from build123d import *

# Parameters (mm, degrees)
F0_W     = 30
F0_H     = 30
F0_W_2   = 25.6
F0_H_2   = 25.6
F1_DEPTH = 200
F2_R     = 3.1
F3_DEPTH = 35
F4_R     = 3.1
F5_DEPTH = 35


with BuildPart() as f1:
    # F0 (on Front) → F1 (new body)
    with BuildSketch(Plane.XZ):
        with Locations((15, 15)):
            Rectangle(F0_W, F0_H)
        with Locations((15, 15)):
            Rectangle(F0_W_2, F0_H_2, mode=Mode.SUBTRACT)
    extrude(amount=F1_DEPTH)

    # F2 (on face) → F3 (cut)
    with BuildSketch(Plane.XY.offset(30)):
        with Locations((15, -20)):
            Circle(F2_R)
        with Locations((15, -100)):
            Circle(F2_R)
        with Locations((15, -180)):
            Circle(F2_R)
    extrude(amount=-F3_DEPTH, mode=Mode.SUBTRACT)

    # F4 (on face) → F5 (cut)
    with BuildSketch(Plane.YZ.offset(30)):
        with Locations((-166.5, 15)):
            Circle(F4_R)
        with Locations((-33.5, 15)):
            Circle(F4_R)
    extrude(amount=-F5_DEPTH, mode=Mode.SUBTRACT)


solid = f1.part
Work out the finished part from the listing and answer in its coordinate system (mm). A direction names the side the tool comes from. Coordinates: 2 decimals unless noted, no trailing zeros. Write each loop counter-clockwise with the first axis right and the second up, starting at its lowest first coordinate (ties: lowest second). Pieces come first, ordered by that corner, then holes. Notation, with made-up numbers: M -14,-20.5 L 21,-20.5 A31 cw 21,18.5 Z; hole C 86,18.5 d2. An arc over 180 degrees is marked long. Use one line per item in the form item = value. Start each with the question number.
1. The part is cut by section C-C (y = -143). Give the vertices of the cut face in (x, z).
2. The part is cut by section D-D (x = 15). Give the number of separate pieces and of enclosed holes in the cut face, plus the area to 3 significant figures.
3. A tool of negligible diameter and unlimited length cuts with its end or side. For faces 4 (the face through (28.915, -163.543, 15.931)), 5 (the face through (12, -98.6, 27.8)), from which of +Z, -Z, +X, -X, +Y, -Y can it reach the whole face along a straight path? Write none if from no direction.
4. The part is cut by section B-B (z = 21). Give the vertices of the cut face in (x, y), plus the area to 3 significant figures.
5. Straight lines are drawn through the part: probe 1 along Y at (x, z) = (15, 29.55); probe 2 along X at (y, z) = (-26, 25.25); probe 3 along X at (y, z) = (-180, 29.55). For each, find the intervals that lie inside material, in ascending order. Write a range as from..to.
6. The part is cut by section A-A (x = 5). Give the vertices of the cut face in (y, z).
7. The mould has two halves that part along X. Classify faces 1 (the face through (14.328, -103.026, 28.915)), 2 (the face through (28, 0, 15)), 3 (the face through (30, -99, 15)): released by +X, released by -X, zero draft, split by the parting line, or undercut.
Evaluation:
q1.outline = M 0,0 L 30,0 L 30,30 L 0,30 Z; hole M 2.2,2.2 L 27.8,2.2 L 27.8,27.8 L 2.2,27.8 Z
q2.separate_pieces = 8
q2.enclosed_holes = 0
q2.area = 798 mm^2
q3.face_4 = +X, -X
q3.face_5 = +Y, -Y
q4.outline = M 0,-200 L 2.2,-200 L 2.2,0 L 0,0 Z; M 27.8,-200 L 30,-200 L 30,0 L 27.8,0 Z
q4.area = 880 mm^2
q5.probe_1 = -200..-183.1, -176.9..-103.1, -96.9..-23.1, -16.9..0
q5.probe_2 = 0..2.2, 27.8..30
q5.probe_3 = 0..11.9, 18.1..30
q6.outline = M -200,0 L 0,0 L 0,2.2 L -200,2.2 Z; M -200,27.8 L 0,27.8 L 0,30 L -200,30 Z
q7.face_1 = undercut
q7.face_2 = zero draft
q7.face_3 = released by +X
